from build123d import *

# Parameters (mm, degrees)
BOSS_EXTRUDE1_DEPTH     = 3
SKETCH1_7_R             = 0.5
BOSS_EXTRUDE2_DEPTH     = 2
BOSS_EXTRUDE4_REACH     = 44.227
SKETCH4_W               = 3
SKETCH4_H               = 12
BOSS_EXTRUDE5_DEPTH     = 5
FILLET3_R               = 10
BOSS_EXTRUDE11_START    = -17
BOSS_EXTRUDE11_DEPTH    = 32.8
SKETCH12_R              = 1
SKETCH12_W              = 12
SKETCH12_H              = 23
CUT_EXTRUDE2_DEPTH      = 48.02396982
FILLET7_R               = 6
FILLET8_R               = 6
SKETCH13_W              = 3
SKETCH13_H              = 10
BOSS_EXTRUDE12_DEPTH    = 2
FILLET9_R               = 5
BOSS_EXTRUDE13_START    = -8
SKETCH1_9_R             = 3
SKETCH1_9_R_2           = 2
BOSS_EXTRUDE13_DEPTH    = 8
CUT_EXTRUDE3_DEPTH      = 8
CUT_EXTRUDE3_DEPTH_BACK = 8
SKETCH1_10_R            = 2
SKETCH1_10_R_2          = 1.15
BOSS_EXTRUDE14_START    = -1
SKETCH1_11_R            = 2
BOSS_EXTRUDE14_DEPTH    = 1
SKETCH1_12_R            = 3
CUT_EXTRUDE4_DEPTH      = 5
SKETCH1_13_R            = 1.15
CUT_EXTRUDE5_DEPTH      = 5
SKETCH17_W              = 11.286302552
SKETCH17_H              = 6
CUT_EXTRUDE6_DEPTH      = 6
BOSS_EXTRUDE15_START    = -3.840535
SKETCH18_W              = 2.041960109
SKETCH18_H              = 1
BOSS_EXTRUDE15_DEPTH    = 3.840535


# Read off the part's stored shape, not the designer's step: Boss-Extrude11
# Some blends are built 0.0001 mm under size
with BuildPart() as part:
    # Sketch1 → Boss-Extrude1 (new body)
    with BuildSketch(Plane(origin=(0, 0, 0), x_dir=(1, 0, 0), z_dir=(0, 1, 0))):
        with BuildLine():
            Line((40.375241408, 5.866153579), (0.375241408, 5.866153579))
            Line((0.375241408, 5.866153579), (0.375241408, 2.102221557))
            ThreePointArc((0.375241408, 2.102221557), (1.113854196, 1.090898451), (1.375241408, -0.133846421))
            ThreePointArc((1.375241408, -0.133846421), (1.113854196, -1.358591292), (0.375241408, -2.369914398))
            Line((0.375241408, -2.369914398), (0.375241408, -6.133846421))
            Line((0.375241408, -6.133846421), (40.375241408, -6.133846421))
            Line((40.375241408, -6.133846421), (40.375241408, 5.866153579))
        make_face()
        with BuildLine():
            Line((32.622415803, -2.8), (20.221989119, -2.1))
            ThreePointArc((20.221989119, -2.1), (18.237190195, 0), (20.221989119, 2.1))
            Line((20.221989119, 2.1), (32.622415803, 2.8))
            ThreePointArc((32.622415803, 2.8), (36.374444489, 3.199023384), (38.375241408, 0))
            ThreePointArc((38.375241408, 0), (36.374444489, -3.199023384), (32.622415803, -2.8))
        make_face(mode=Mode.SUBTRACT)
    extrude(amount=BOSS_EXTRUDE1_DEPTH)

    # Sketch1<7> → Boss-Extrude2 (add)
    with BuildSketch(Plane(origin=(0, 0, 0), x_dir=(1, 0, 0), z_dir=(0, 1, 0))):
        with BuildLine():
            ThreePointArc((20.221989119, 2.1), (18.237190195, 0), (20.221989119, -2.1))
            Line((20.221989119, -2.1), (32.622415803, -2.8))
            ThreePointArc((32.622415803, -2.8), (31.259607239, 0), (32.622415803, 2.8))
            Line((32.622415803, 2.8), (20.221989119, 2.1))
        make_face()
        with Locations(Location((20.005781193, 0, 0), (0, 0, 270))):
            Circle(SKETCH1_7_R, mode=Mode.SUBTRACT)
        with Locations(Location((22.005781193, 0, 0), (0, 0, 270))):
            Circle(SKETCH1_7_R, mode=Mode.SUBTRACT)
        with Locations(Location((24.005781193, 0, 0), (0, 0, 270))):
            Circle(SKETCH1_7_R, mode=Mode.SUBTRACT)
        with Locations(Location((26.005781193, 0, 0), (0, 0, 270))):
            Circle(SKETCH1_7_R, mode=Mode.SUBTRACT)
        with Locations(Location((28.005781193, 0, 0), (0, 0, 270))):
            Circle(SKETCH1_7_R, mode=Mode.SUBTRACT)
        with Locations(Location((30.005781193, 0, 0), (0, 0, 270))):
            Circle(SKETCH1_7_R, mode=Mode.SUBTRACT)
    extrude(amount=BOSS_EXTRUDE2_DEPTH)

    # Boss-Extrude4: up to this face of the body (flat: up to its plane)
    boss_extrude4_end = Plane(part.part.faces().sort_by_distance((20.375241408, 1.5, -5.866153579))[0])
    # Sketch3 → Boss-Extrude4 (add, up to the picked face)
    with BuildSketch(Plane.XY.offset(6.133846421), mode=Mode.PRIVATE) as boss_extrude4_sk1:
        Polygon((0.375241408, 3), (-9.624758592, -4), (-4.393377613, -4), (5.606622387, 3), align=None)
    boss_extrude4_tool1 = split(extrude(boss_extrude4_sk1.sketch, amount=-BOSS_EXTRUDE4_REACH, mode=Mode.PRIVATE), bisect_by=boss_extrude4_end, keep=Keep.BOTH, mode=Mode.PRIVATE)
    add(boss_extrude4_tool1.solids().sort_by(Axis((-2.009068, -0.5, 6.133846), (0, 0, -1)))[0])

    # Sketch4 → Boss-Extrude5 (add)
    with BuildSketch(Plane(origin=(0, -4, 0), x_dir=(-1, 0, 0), z_dir=(0, -1, 0))):
        with Locations((8.124758592, -0.133846421)):
            Rectangle(SKETCH4_W, SKETCH4_H)
    extrude(amount=BOSS_EXTRUDE5_DEPTH)

    # Fillet3
    # the kernel refuses this fillet: 10 mm, written as the material it adds along each edge
    with BuildSketch(Plane(origin=(1.320908101, 0, 6.133846421), x_dir=(1, 0, 0), z_dir=(0, 0, -1))) as fillet3_piece_1_section:
        with BuildLine():
            CenterArc((FILLET3_R * 0.315222230819, FILLET3_R), FILLET3_R, 235.007979801, 34.992020199)
            Line((-FILLET3_R * 0.258240113544, FILLET3_R * 0.180768079481), (0, 0))
            Line((0, 0), (FILLET3_R * 0.315222230819, 0))
        make_face()
    fillet3_piece_1 = extrude(amount=13.312182885, mode=Mode.PRIVATE)
    fillet3_piece_1 = split(fillet3_piece_1, bisect_by=Plane(origin=(1.586628452, -0.313093782, -5.866153579), z_dir=(0, 0, 1)), keep=Keep.TOP, mode=Mode.PRIVATE)
    fillet3_piece_1 = fillet3_piece_1 - Plane(origin=(-1.624758592, -0.313093782, 0.133846421), x_dir=(0.6666666666666657, 0, -0.7453559924999308), z_dir=(0, -1, 0)) * Cylinder(3, 40, mode=Mode.PRIVATE)
    add(fillet3_piece_1)
    with BuildSketch(Plane(origin=(1.320908101, 0, 7.446029306), x_dir=(1, 0, 0), z_dir=(0, 0, -1))) as fillet3_piece_2_section:
        with BuildLine():
            CenterArc((FILLET3_R * 0.315222230819, FILLET3_R), FILLET3_R, 235.007979801, 34.992020199)
            Line((-FILLET3_R * 0.258240113544, FILLET3_R * 0.180768079481), (0, 0))
            Line((0, 0), (FILLET3_R * 0.315222230819, 0))
        make_face()
    fillet3_piece_2 = extrude(amount=13.312182885, mode=Mode.PRIVATE)
    fillet3_piece_2 = split(fillet3_piece_2, bisect_by=Plane(origin=(1.586628452, -0.313093782, 6.133846421), z_dir=(0, 0, -1)), keep=Keep.TOP, mode=Mode.PRIVATE)
    fillet3_piece_2 = fillet3_piece_2 - Plane(origin=(-1.624758592, -0.313093782, 0.133846421), x_dir=(0.6666666666666657, 0, -0.7453559924999308), z_dir=(0, -1, 0)) * Cylinder(3, 40, mode=Mode.PRIVATE)
    add(fillet3_piece_2)

    # Boss-Extrude11 outline → Boss-Extrude11 (add)
    with BuildSketch(Plane.XY.offset(6.133846421).offset(BOSS_EXTRUDE11_START)):
        Polygon((-9.624758592, -7), (-9.624758592, -9), (-6.624758592, -9), (-6.624758592, -4), (-24.624758592, -4), (-24.624758592, -7), align=None)
    extrude(amount=BOSS_EXTRUDE11_DEPTH)

    # Sketch12 → Cut-Extrude2 (cut, through all)
    with BuildSketch(Plane(origin=(0, -7, 0), x_dir=(-1, 0, 0), z_dir=(0, -1, 0))):
        with Locations(Location((15.624758592, -19.133846421, 0), (0, 0, 180))):
            Circle(SKETCH12_R)
        with Locations(Location((15.624758592, 7.866153579, 0), (0, 0, 180))):
            Circle(SKETCH12_R)
        with Locations((15.624758592, -5.633846421)):
            Rectangle(SKETCH12_W, SKETCH12_H)
    extrude(amount=-CUT_EXTRUDE2_DEPTH, mode=Mode.SUBTRACT)

    # Fillet7
    fillet7_edges = [part.edges().sort_by_distance(p)[0] for p in [
        (40.375241408, 1.5, -5.866153579),
        (40.375241408, 1.5, 6.133846421),
    ]]
    fillet(fillet7_edges, radius=FILLET7_R - 0.0001)  # a hair under: the kernel refuses the full size

    # Fillet8
    # the kernel refuses this fillet: 6 mm, written as the material it adds along each edge
    with BuildSketch(Plane(origin=(-6.624758592, -4, -5.866153579), x_dir=(1, 0, 0), z_dir=(0, 0, 1))) as fillet8_piece_1:
        with BuildLine():
            CenterArc((6, -4.668780426), FILLET8_R, 128.910316117, 51.089683883)
            Line((0, -4.668780426), (0, 0))
            Line((0, 0), (2.231380978, 0))
        make_face()
    extrude(amount=12)

    # Sketch13 → Boss-Extrude12 (add)
    with BuildSketch(Plane.XZ.offset(7)):
        with Locations((-23.124758592, 5.633846421)):
            Rectangle(SKETCH13_W, SKETCH13_H)
    extrude(amount=BOSS_EXTRUDE12_DEPTH)

    # Fillet9
    # the kernel refuses this fillet: 5 mm, written as the material it takes off along each edge
    with BuildSketch(Plane(origin=(-6.624758592, -21.5, -10.866153579), x_dir=(0, 0, 1), z_dir=(0, 1, 0))) as fillet9_piece_1:
        with BuildLine():
            CenterArc((FILLET9_R, -FILLET9_R), FILLET9_R, 90, 90)
            Line((0, -FILLET9_R), (0, 0))
            Line((0, 0), (FILLET9_R, 0))
        make_face()
    extrude(amount=30, mode=Mode.SUBTRACT)
    with BuildSketch(Plane(origin=(-24.624758592, 8.5, -10.866153579), x_dir=(1, 0, 0), z_dir=(0, -1, 0))) as fillet9_piece_2:
        with BuildLine():
            CenterArc((FILLET9_R, FILLET9_R), FILLET9_R, 180, 90)
            Line((0, FILLET9_R), (0, 0))
            Line((0, 0), (FILLET9_R, 0))
        make_face()
    extrude(amount=28, mode=Mode.SUBTRACT)
    with BuildSketch(Plane(origin=(-24.624758592, 8.5, 21.933846421), x_dir=(1, 0, 0), z_dir=(0, -1, 0))) as fillet9_piece_3:
        with BuildLine():
            CenterArc((FILLET9_R, -FILLET9_R), FILLET9_R, 90, 90)
            Line((0, -FILLET9_R), (0, 0))
            Line((0, 0), (FILLET9_R, 0))
        make_face()
    extrude(amount=28, mode=Mode.SUBTRACT)
    with BuildSketch(Plane(origin=(-6.624758592, -21.5, 21.933846421), x_dir=(0, 0, -1), z_dir=(0, 1, 0))) as fillet9_piece_4:
        with BuildLine():
            CenterArc((FILLET9_R, FILLET9_R), FILLET9_R, 180, 90)
            Line((0, FILLET9_R), (0, 0))
            Line((0, 0), (FILLET9_R, 0))
        make_face()
    extrude(amount=30, mode=Mode.SUBTRACT)

    # Sketch1<9> → Boss-Extrude13 (add)
    with BuildSketch(Plane(origin=(0, 0, 0), x_dir=(1, 0, 0), z_dir=(0, 1, 0)).offset(BOSS_EXTRUDE13_START)):
        with Locations(Location((-1.624758592, -0.133846421, 0), (0, 0, 270))):
            Circle(SKETCH1_9_R)
        with Locations(Location((-1.624758592, -0.133846421, 0), (0, 0, 270))):
            Circle(SKETCH1_9_R_2, mode=Mode.SUBTRACT)
    extrude(amount=BOSS_EXTRUDE13_DEPTH)

    # Sketch1<10> → Cut-Extrude3 (cut, two sides: drawn at the far end of the back side and taken through both)
    with BuildSketch(Plane(origin=(0, 0, 0), x_dir=(1, 0, 0), z_dir=(0, 1, 0)).offset(-CUT_EXTRUDE3_DEPTH_BACK)):
        with Locations(Location((-1.624758592, -0.133846421, 0), (0, 0, 270))):
            Circle(SKETCH1_10_R)
        with Locations((-1.624758592, -0.133846421)):
            Circle(SKETCH1_10_R_2)
    extrude(amount=CUT_EXTRUDE3_DEPTH + CUT_EXTRUDE3_DEPTH_BACK, mode=Mode.SUBTRACT)

    # Sketch1<11> → Boss-Extrude14 (add)
    with BuildSketch(Plane(origin=(0, 0, 0), x_dir=(1, 0, 0), z_dir=(0, 1, 0)).offset(BOSS_EXTRUDE14_START)):
        with Locations(Location((-1.624758592, -0.133846421, 0), (0, 0, 270))):
            Circle(SKETCH1_11_R)
    extrude(amount=BOSS_EXTRUDE14_DEPTH)

    # Sketch1<12> → Cut-Extrude4 (cut)
    with BuildSketch(Plane(origin=(0, 0, 0), x_dir=(1, 0, 0), z_dir=(0, 1, 0))):
        with Locations(Location((-1.624758592, -0.133846421, 0), (0, 0, 270))):
            Circle(SKETCH1_12_R)
    extrude(amount=CUT_EXTRUDE4_DEPTH, mode=Mode.SUBTRACT)

    # Sketch1<13> → Cut-Extrude5 (cut)
    with BuildSketch(Plane(origin=(0, 0, 0), x_dir=(1, 0, 0), z_dir=(0, 1, 0))):
        with Locations(Location((-1.624758592, -0.133846421, 0), (0, 0, 270))):
            Circle(SKETCH1_13_R)
    extrude(amount=-CUT_EXTRUDE5_DEPTH, mode=Mode.SUBTRACT)

    # Sketch17 → Cut-Extrude6 (cut)
    with BuildSketch(Plane(origin=(0, 0, 0), x_dir=(1, 0, 0), z_dir=(0, 1, 0))):
        with Locations((-7.267909868, -0.133846421)):
            Rectangle(SKETCH17_W, SKETCH17_H)
    extrude(amount=CUT_EXTRUDE6_DEPTH, mode=Mode.SUBTRACT)

    # Sketch18 → Boss-Extrude15 (add)
    with BuildSketch(Plane(origin=(0, -8, 0), x_dir=(-1, 0, 0), z_dir=(0, -1, 0)).offset(BOSS_EXTRUDE15_START)):
        with Locations((5.603778538, -0.133846421)):
            Rectangle(SKETCH18_W, SKETCH18_H)
    extrude(amount=BOSS_EXTRUDE15_DEPTH)


solid = part.part
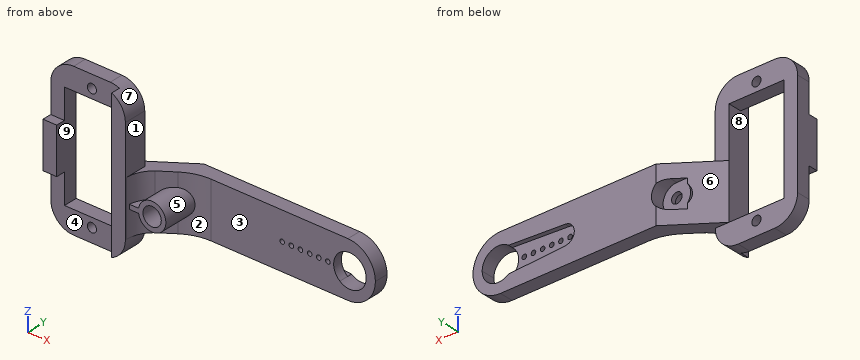
Verification items for the finished model (mm, model axes). Face numbers are marked on the shaded views. A direction names the side the tool comes from. Give positions to 0.01 mm unless a question says otherwise; leave off trailing zeros. Write each loop counter-clockwise with the first axis right and the second up, starting at its lowest first coordinate (ties: lowest second). Pieces come first, ordered by that corner, then holes. Notation, with made-up numbers: (-12, -5.75) -> (-2, -5.75) arc R19 cw to (-2, 19.25) -> close; hole circle Ø7 at (81, 24.5). An arc over 180 degrees is marked (long way). Use CSV: the item, a comma, the result in double quotes.
(1) Set-up check for the marked faces 1, 2, 3, 4 and 5: record each of +Z, -Z, +X, -X, +Y, -Y from which the full face is reachable in a straight line by a thin tool's end or side.
Derived:
face 1,"+Z, +X, -Y"
face 2,"+X, -Y"
face 3,"+Z, -Z, +X, -Y"
face 4,"-Z, -X, -Y"
face 5,"-Y"
(2) Go/stop test with flat-tipped pins: pin 1 (0.6 mm diameter, centred on x = -22.5, y = -8, fed in from -Z); pin 2 (4 mm diameter, centred on x = 13.5, z = 5.5, fed in from -Y); pin 3 (6 mm diameter, centred on x = 7, y = -1.5, fed in from +Z). Record where each tip stops, or that it passes through.
Derived:
pin 1,"stops at z = 0.63"
pin 2,"stops at y = 0"
pin 3,"stops at z = 6.13"
(3) Sectioned sample at B-B (y = -6). Record the cut outline in (x, z), plus the area to 3 significant figures.
Derived:
outline,"(-24.62, -5.87) arc R5 ccw to (-19.62, -10.87) -> (-11.62, -10.87) arc R5 ccw to (-6.62, -5.87) -> (-6, -5.87) -> (-6, -0.37) -> (-4.58, -0.37) arc R3 ccw (long way) to (-4.58, 0.63) -> (-6, 0.63) -> (-6, 6.13) -> (-6.62, 6.13) -> (-6.62, 16.93) arc R5 ccw to (-11.62, 21.93) -> (-19.62, 21.93) arc R5 ccw to (-24.62, 16.93) -> close; hole (-21.62, -5.87) -> (-9.62, -5.87) -> (-9.62, 17.13) -> (-21.62, 17.13) -> close; hole circle Ø2 at (-15.62, -7.87); hole circle Ø2 at (-15.62, 19.13); hole circle Ø4 at (-1.62, 0.13)"
area,"311 mm^2"
(4) Sectioned sample at A-A (z = 13). Record the cut outline in (x, y).
Derived:
outline,"(-24.62, -7) -> (-21.62, -7) -> (-21.62, -4) -> (-24.62, -4) -> close; (-9.62, -9) -> (-6.62, -9) -> (-6.62, -4) -> (-9.62, -4) -> close"
(5) Release check for a two-part mould opening along Z. For the marked faces 6, 7, 8 and 9 record: +Z half, -Z half, draft (parallel to the pull), parting line (faces both ways), or undercut.
Derived:
face 6,"draft"
face 7,"+Z half"
face 8,"undercut"
face 9,"undercut"
(6) Sectioned sample at C-C (x = 16). Record the cut outline in (y, z).
Derived:
outline,"(0, -5.87) -> (3, -5.87) -> (3, 6.13) -> (0, 6.13) -> close"
(7) Material ranges on L1, parallel to X at y = -7.75, z = 8; L2, parallel to Y at x = -17.5, z = -8.5; L3, parallel to Z at x = -12, y = -6.25, recorded low to high.
Derived:
L1,"x = -24.62 to -21.62, -9.62 to -6.62"
L2,"y = -7 to -4"
L3,"z = -10.87 to -5.87, 17.13 to 21.93"
